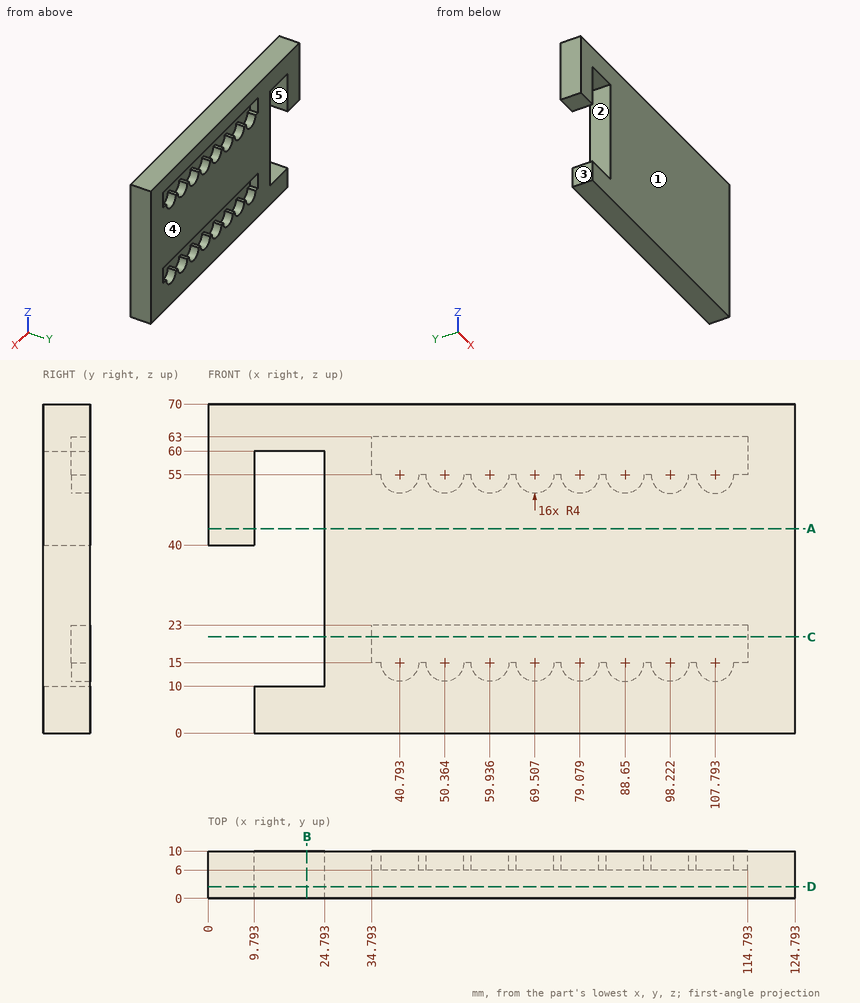
Study the drawing (mm; zero at the part's minimum x, y, z) and answer. A direction names the side the tool comes from. Round coordinates to 2 decimals unless told otherwise and drop trailing zeros. Write each loop counter-clockwise with the first axis right and the second up, starting at its lowest first coordinate (ties: lowest second). Pieces come first, ordered by that corner, then holes.
1) A cutting plane is placed at C-C (z = 20.5). Give the vertices of the cut face in (x, y).
2) A tool of negligible diameter and unlimited length cuts with its end or side. For the marked faces 1 and 2, from which of +Z, -Z, +X, -X, +Y, -Y can it reach the whole face along a straight path? Write none if from no direction.
3) The mould has two halves that part along X. Classify the marked faces 3, 4 and 5: pulls with the +X half, pulls with the -X half, needs draft (parallel to the pull), parting line crosses it, or undercut.
4) A cutting plane is placed at D-D (y = 2.5). Give the vertices of the cut face in (x, z).
5) A cutting plane is placed at A-A (z = 43.5). Give the vertices of the cut face in (x, y), plus the area to 3 significant figures.
6) A cutting plane is placed at B-B (x = 21). Give the vertices of the cut face in (y, z), plus the area to 3 significant figures.
7) Given pin 1 Ø1.5 at (y, z) = (6, 23.5) entering from -X, flat-ended and moving along its own axis, determine where the tip first touches the part or whether it passes through.
8) Straight lines are drawn through the part: line 1 (Z direction, x = 114, y = 9); line 2 (Z direction, x = 14, y = 2.75); line 3 (X direction, y = 7.5, z = 31.5). For each, find the intervals that lie inside material, in ascending order.
Completed:
1. outline: (24.79, 0) - (124.79, 0) - (124.79, 10) - (114.79, 10) - (114.79, 6) - (34.79, 6) - (34.79, 10) - (24.79, 10) - close
2. face 1: +Z, -Z, +X, -X, -Y
2. face 2: +Y, -Y
3. face 3: pulls with the -X half
3. face 4: needs draft
3. face 5: undercut
4. outline: (0, 40) - (9.79, 40) - (9.79, 60) - (24.79, 60) - (24.79, 10) - (9.79, 10) - (9.79, 0) - (124.79, 0) - (124.79, 70) - (0, 70) - close
5. outline: (0, 0) - (9.79, 0) - (9.79, 10) - (0, 10) - close; (24.79, 0) - (124.79, 0) - (124.79, 10) - (24.79, 10) - close
5. area: 1,100 mm2
6. outline: (0, 0) - (10, 0) - (10, 10) - (0, 10) - close; (0, 60) - (10, 60) - (10, 70) - (0, 70) - close
6. area: 200 mm2
7. pin 1: stops at x = 24.79
8. line 1: z = 0 to 15, 23 to 55, 63 to 70
8. line 2: z = 0 to 10, 60 to 70
8. line 3: x = 24.79 to 124.79
